```python
from build123d import *

# Parameters (mm, degrees)
AUFSATZ_LINEAR_AUSTRAGEN1_DEPTH = 25
SKIZZE2_W                       = 3
SKIZZE2_H                       = 4
SCHNITT_LINEAR_AUSTRAGEN1_DEPTH = 25
SKIZZE3_R                       = 9.5
SCHNITT_LINEAR_AUSTRAGEN2_DEPTH = 35
SKIZZE4_R                       = 11
SCHNITT_LINEAR_AUSTRAGEN3_DEPTH = 6
SKIZZE5_R                       = 11
SCHNITT_LINEAR_AUSTRAGEN4_DEPTH = 6


with BuildPart() as part:
    # Skizze1 → Aufsatz-Linear austragen1 (new body)
    with BuildSketch(Plane(origin=(0, 0, 0), x_dir=(1, 0, 0), z_dir=(0, 1, 0))):
        Polygon((-8, 0), (-8, 26), (-16, 26), (-16, -4), (16, -4), (16, 26), (8, 26), (8, 0), align=None)
    extrude(amount=AUFSATZ_LINEAR_AUSTRAGEN1_DEPTH)

    # Skizze2 → Schnitt-Linear austragen1 (cut)
    with BuildSketch(Plane.XZ):
        with Locations((14.5, -1)):
            Rectangle(SKIZZE2_W, SKIZZE2_H)
        with Locations((-14.5, -1)):
            Rectangle(SKIZZE2_W, SKIZZE2_H)
    extrude(amount=-SCHNITT_LINEAR_AUSTRAGEN1_DEPTH, mode=Mode.SUBTRACT)

    # Skizze3 → Schnitt-Linear austragen2 (cut)
    with BuildSketch(Plane.ZY.offset(16)):
        with Locations((-14.5, 12.5)):
            Circle(SKIZZE3_R)
    extrude(amount=-SCHNITT_LINEAR_AUSTRAGEN2_DEPTH, mode=Mode.SUBTRACT)

    # Skizze4 → Schnitt-Linear austragen3 (cut)
    with BuildSketch(Plane.ZY.offset(16)):
        with Locations((-14.5, 12.5)):
            Circle(SKIZZE4_R)
    extrude(amount=-SCHNITT_LINEAR_AUSTRAGEN3_DEPTH, mode=Mode.SUBTRACT)

    # Skizze5 → Schnitt-Linear austragen4 (cut)
    with BuildSketch(Plane(origin=(16, 0, 0), x_dir=(0, 0, -1), z_dir=(1, 0, 0))):
        with Locations((14.5, 12.5)):
            Circle(SKIZZE5_R)
    extrude(amount=-SCHNITT_LINEAR_AUSTRAGEN4_DEPTH, mode=Mode.SUBTRACT)


solid = part.part
```
For this review, take the finished solid that the model builds, in its own axes (mm). A direction names the side the tool comes from. Round coordinates to 2 decimals unless told otherwise and drop trailing zeros. Write each loop counter-clockwise with the first axis right and the second up, starting at its lowest first coordinate (ties: lowest second). Pieces come first, ordered by that corner, then holes.
1) For line 1 along Y through (x, z) = (8.9, -14.5); line 2 along X through (y, z) = (19, -7.5); line 3 along Y through (x, z) = (13, -14.5), list the stretches that pass through material, from the lowest coordinate up.
Answer below:
line 1: y = 0 to 3, 22 to 25
line 2: x = -10 to -8, 8 to 10
line 3: y = 0 to 1.5, 23.5 to 25
2) Take a section at A-A on z = -14.5. Give the boundary of the cut face in (x, y), then the cut area to 3 significant figures.
Answer below:
outline: (-16, 0) - (-8, 0) - (-8, 3) - (-10, 3) - (-10, 1.5) - (-16, 1.5) - close; (-16, 23.5) - (-10, 23.5) - (-10, 22) - (-8, 22) - (-8, 25) - (-16, 25) - close; (8, 0) - (16, 0) - (16, 1.5) - (10, 1.5) - (10, 3) - (8, 3) - close; (8, 22) - (10, 22) - (10, 23.5) - (16, 23.5) - (16, 25) - (8, 25) - close
area: 60.0 mm2
3) Take a section at B-B on y = 12.5. State how many separate pieces and enclosed holes the cut face has, then the cut area to 3 significant figures.
Answer below:
separate pieces: 3
enclosed holes: 0
area: 180 mm2
4) Take a section at D-D on x = 12.5. Give the boundary of the cut face in (y, z).
Answer below:
outline: (0, -26) - (25, -26) - (25, 4) - (0, 4) - close; hole circle Ø22 at (12.5, -14.5)
5) Mouldability with a two-part tool opening along Z and no side actions: class faces 1 (the face through (-8, 12, -4)), 2 (the face through (13.04, 1.76, -12.12)), 3 (the face through (12, 12, -26)) as +Z half, -Z half, draft (parallel to the pull), parting line (faces both ways), or undercut.
Answer below:
face 1: draft
face 2: undercut
face 3: -Z half
6) Take a section at C-C on z = -2.25. Give the boundary of the cut face in (x, y).
Answer below:
outline: (-13, 0) - (-8, 0) - (-8, 25) - (-13, 25) - close; (8, 0) - (13, 0) - (13, 25) - (8, 25) - close
7) Machinability: for faces 4 (the face through (-15, 12, -3)), 5 (the face through (10, 9, -5)), 6 (the face through (14, 12, 1)), 7 (the face through (-13.042, 2.741, -9.424)), which of the approach directions +Z, -Z, +X, -X, +Y, -Y give a long, thin tool a straight path to every point of the face, cutting with its end or side? Answer none if there is none.
Answer below:
face 4: -X, +Y, -Y
face 5: +X
face 6: +X, +Y, -Y
face 7: -X
8) Insertion check: pin 1 Ø1.2 at (y, z) = (18.5, 0) entering from -X; pin 2 Ø6 at (x, y) = (-0.5, 12.5) entering from -Z. Each pin has a flat end and moves straight along its axis. Give the tip position at first contact, or say it passes through.
Answer below:
pin 1: stops at x = -13
pin 2: stops at z = 0
